Verification items for this drawing (mm, ordinates from the low corner). A direction names the side the tool comes from. Coordinates: 2 decimals unless noted, no trailing zeros. Order: outer loops, then holes, each group sorted by start corner. A loop starts at its lowest first (then second) coordinate and runs counter-clockwise, first axis right, second up.
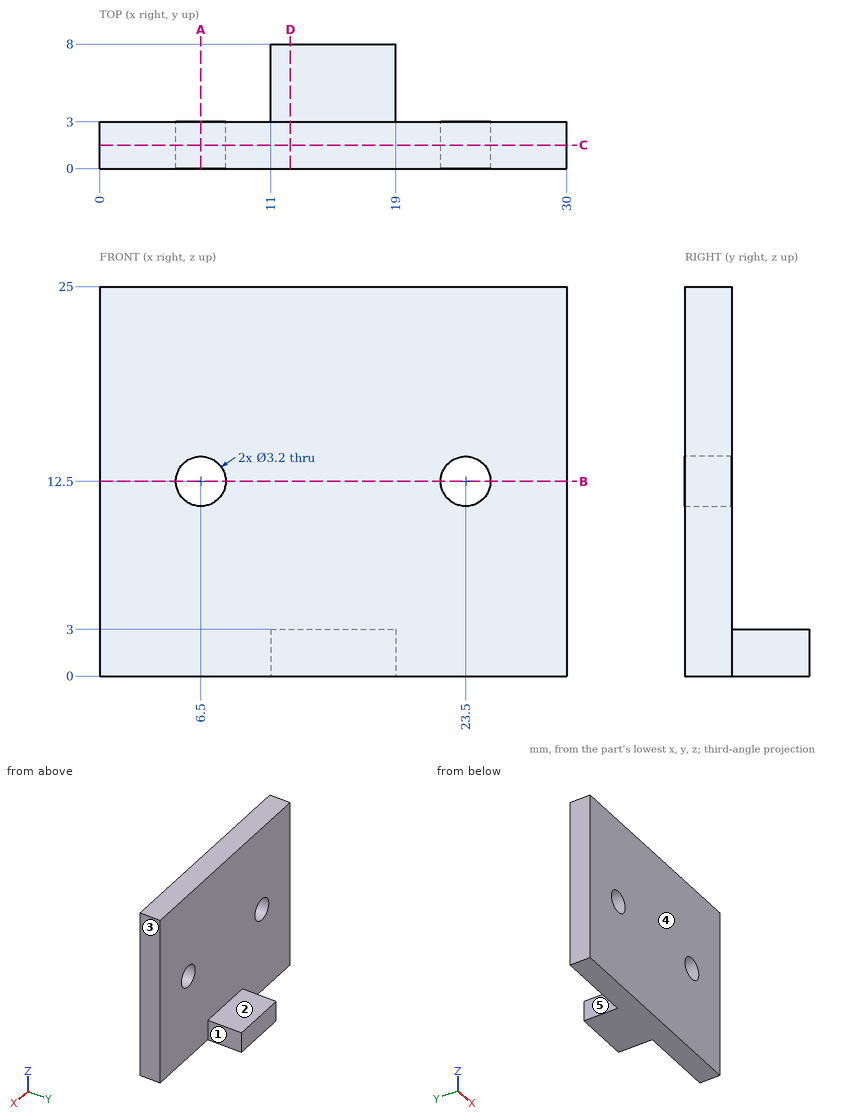
(1) Cross-section at D-D (x = 12.25). Enter the section's corners in (y, z), and give its area (3 significant figures).
Filled in:
outline: (0, 0) - (8, 0) - (8, 3) - (3, 3) - (3, 25) - (0, 25) - close
area: 90.0 mm2
(2) Thickness scan on probe 1 along X at (y, z) = (1.65, 12.5); probe 2 along X at (y, z) = (1.75, 11.5); probe 3 along Y at (x, z) = (19.5, 19). Record the ranges inside material, lowest first.
Filled in:
probe 1: x = 0 to 4.9, 8.1 to 21.9, 25.1 to 30
probe 2: x = 0 to 5.25, 7.75 to 22.25, 24.75 to 30
probe 3: y = 0 to 3
(3) Cross-section at A-A (x = 6.5). Enter the section's corners in (y, z).
Filled in:
outline: (0, 0) - (3, 0) - (3, 10.9) - (0, 10.9) - close; (0, 14.1) - (3, 14.1) - (3, 25) - (0, 25) - close
(4) Go/stop test with flat-tipped pins: P1, Ø1.5, axis at x = 16, y = 5.5, coming from the +Z side; P2, Ø0.9, axis at y = 6, z = 1.5, coming from the +X side; P3, Ø3.5, axis at x = 6.5, z = 12.5, coming from the +Y side. Record where each tip stops, or that it passes through.
Filled in:
P1: stops at z = 3
P2: stops at x = 19
P3: stops at y = 3
(5) Tool access check on the marked faces 1, 2, 3, 4 and 5. Record the directions out of +Z, -Z, +X, -X, +Y, -Y that give a thin tool (end or side, any length) a straight path to the whole face; none if there is none.
Filled in:
face 1: +Z, -Z, +X, +Y
face 2: +Z, +X, -X, +Y
face 3: +Z, -Z, +X, +Y, -Y
face 4: +Z, -Z, +X, -X, -Y
face 5: +Z, -Z, -X, +Y
(6) Cross-section at B-B (z = 12.5). Enter the section's corners in (x, y), and give its area (3 significant figures).
Filled in:
outline: (0, 0) - (4.9, 0) - (4.9, 3) - (0, 3) - close; (8.1, 0) - (21.9, 0) - (21.9, 3) - (8.1, 3) - close; (25.1, 0) - (30, 0) - (30, 3) - (25.1, 3) - close
area: 70.8 mm2
(7) Cross-section at C-C (y = 1.5). Enter the section's corners in (x, z), and give its area (3 significant figures).
Filled in:
outline: (0, 0) - (30, 0) - (30, 25) - (0, 25) - close; hole circle Ø3.2 at (6.5, 12.5); hole circle Ø3.2 at (23.5, 12.5)
area: 734 mm2
